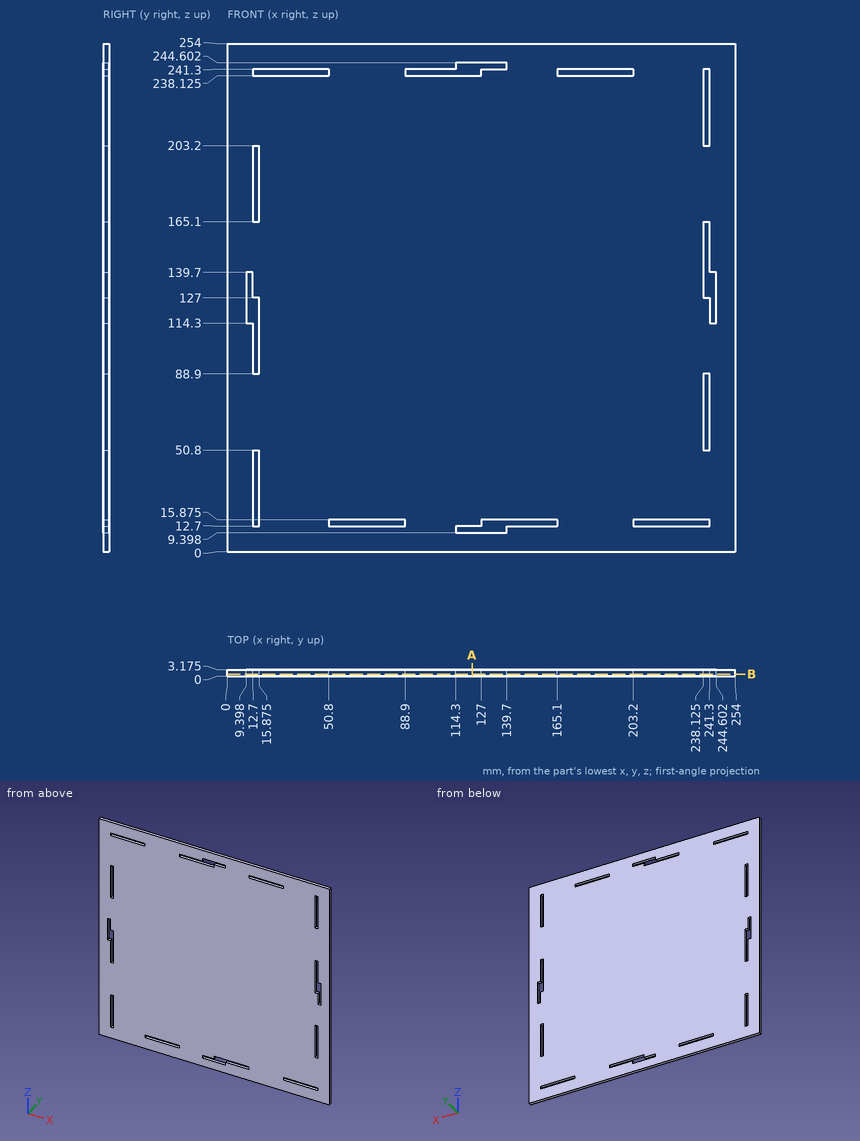
Study the drawing (mm; zero at the part's minimum x, y, z) and answer. Give positions to 0.01 mm unless a question says otherwise; leave off trailing zeros. Order: outer loops, then holes, each group sorted by start corner. A loop starts at its lowest first (then second) coordinate and runs counter-clockwise, first axis right, second up.
1) Find section B-B on y = 0.9. Give the number of separate pieces and of enclosed holes in the cut face, then the cut area to 3 significant figures.
Reported:
separate pieces: 1
enclosed holes: 12
area: 62,700 mm2
2) Find section A-A on x = 122.5. Write down the section's boundary in (y, z) (3 decimals).
Reported:
outline: (0, 0) - (3.175, 0) - (3.175, 9.398) - (0, 9.398) - close; (0, 12.7) - (3.175, 12.7) - (3.175, 238.125) - (0, 238.125) - close; (0, 244.602) - (3.175, 244.602) - (3.175, 254) - (0, 254) - close
3) Consider line 1 along X through (y, z) = (2.35, 129) (3 decimals); line 2 along X through (y, z) = (1.6, 238.5) (3 decimals). Determine where each line is inside the solid, lowest interval first.
Reported:
line 1: x = 0 to 9.398, 12.7 to 238.125, 244.602 to 254
line 2: x = 0 to 12.7, 50.8 to 88.9, 127 to 165.1, 203.2 to 238.125, 241.3 to 254
